from build123d import *

# Parameters (mm, degrees)
EXTRUDE_1_DEPTH        = 52
SKETCH_2_W             = 14.5
SKETCH_2_H             = 8
CUT_EXTRUDE_1_DEPTH    = 4
PATTERN_LINEAR_1_COUNT = 5
PATTERN_LINEAR_1_PITCH = 10
CUT_EXTRUDE_2_DEPTH    = 6.5
PATTERN_LINEAR_2_COUNT = 5
PATTERN_LINEAR_2_PITCH = 10
SKETCH_5_W             = 3
SKETCH_5_H             = 2
SKETCH_5_W_2           = 2
SKETCH_5_H_2           = 1
CUT_EXTRUDE_3_DEPTH    = 3
PATTERN_LINEAR_3_COUNT = 6
PATTERN_LINEAR_3_PITCH = 10
EXTRUDE_2_DEPTH        = 3.5
SKETCH_8_W             = 2
SKETCH_8_H             = 0.5
CUT_EXTRUDE_4_DEPTH    = 5


with BuildPart() as part:
    # 草图1 → 凸台-拉伸1 (new body)
    with BuildSketch(Plane(origin=(0, 0, 0), x_dir=(1, 0, 0), z_dir=(0, 1, 0))):
        Polygon((0, 19), (-2.5, 19), (0, 0), (17.5, 0), (17.5, 3), (3, 3), (3, 19), align=None)
    extrude(amount=EXTRUDE_1_DEPTH)

    # 草图2 → 切除-拉伸1 (cut, through all)
    with BuildSketch(Plane(origin=(0, 0, -3), x_dir=(-1, 0, 0), z_dir=(0, 0, -1))):
        with Locations((-10.25, 46)):
            Rectangle(SKETCH_2_W, SKETCH_2_H)
    cut_extrude_1 = extrude(amount=-CUT_EXTRUDE_1_DEPTH, mode=Mode.SUBTRACT)

    # 阵列(线性)1: 切除-拉伸1 ×5
    with Locations(*[(0, -i * PATTERN_LINEAR_1_PITCH, 0) for i in range(1, PATTERN_LINEAR_1_COUNT)]):
        add(cut_extrude_1, mode=Mode.SUBTRACT)

    # 草图4 → 切除-拉伸2 (cut, through all)
    with BuildSketch(Plane(origin=(3, 0, 0), x_dir=(0, 0, -1), z_dir=(1, 0, 0))):
        Polygon((3, 50), (3, 42), (10, 42.21875), (10, 49.78125), align=None)
        Polygon((19, 49.5), (19, 42.5), (12.5, 42.296875), (12.5, 49.703125), align=None)
    cut_extrude_2 = extrude(amount=-CUT_EXTRUDE_2_DEPTH, mode=Mode.SUBTRACT)

    # 阵列(线性)2: 切除-拉伸2 ×5
    with Locations(*[(0, -i * PATTERN_LINEAR_2_PITCH, 0) for i in range(1, PATTERN_LINEAR_2_COUNT)]):
        add(cut_extrude_2, mode=Mode.SUBTRACT)

    # 草图5 → 切除-拉伸3 (cut)
    with BuildSketch(Plane(origin=(17.5, 0, 0), x_dir=(0, 0, -1), z_dir=(1, 0, 0))):
        with Locations((1.5, 51)):
            Rectangle(SKETCH_5_W, SKETCH_5_H)
        with Locations((1.5, 51)):
            Rectangle(SKETCH_5_W_2, SKETCH_5_H_2, mode=Mode.SUBTRACT)
    cut_extrude_3 = extrude(amount=-CUT_EXTRUDE_3_DEPTH, mode=Mode.SUBTRACT)

    # 阵列(线性)3: 切除-拉伸3 ×6
    with Locations(*[(0, -i * PATTERN_LINEAR_3_PITCH, 0) for i in range(1, PATTERN_LINEAR_3_COUNT)]):
        add(cut_extrude_3, mode=Mode.SUBTRACT)

    # 草图6 → 凸台-拉伸2 (add)
    with BuildSketch(Plane(origin=(3, 0, 0), x_dir=(0, 0, -1), z_dir=(1, 0, 0))):
        Polygon((8.5, 0), (8.5, 0.5), (12.5, 0.5), (12.5, 0), (12.5, -0.5), (8.5, -0.5), align=None)
    extrude_2 = extrude(amount=EXTRUDE_2_DEPTH)

    # 草图8 → 切除-拉伸4 (cut)
    with BuildSketch(Plane.XY.offset(-8.5)):
        with Locations((4, -0.25)):
            Rectangle(SKETCH_8_W, SKETCH_8_H)
        Polygon((6.5, -0.5), (5.1, -0.5), (6.5, 0.2), align=None)
    cut_extrude_4 = extrude(amount=-CUT_EXTRUDE_4_DEPTH, mode=Mode.SUBTRACT)

    # 镜向1: 凸台-拉伸2, 切除-拉伸4 across plane
    add(extrude_2.mirror(Plane.ZX.offset(26)))
    add(cut_extrude_4.mirror(Plane.ZX.offset(26)), mode=Mode.SUBTRACT)


solid = part.part
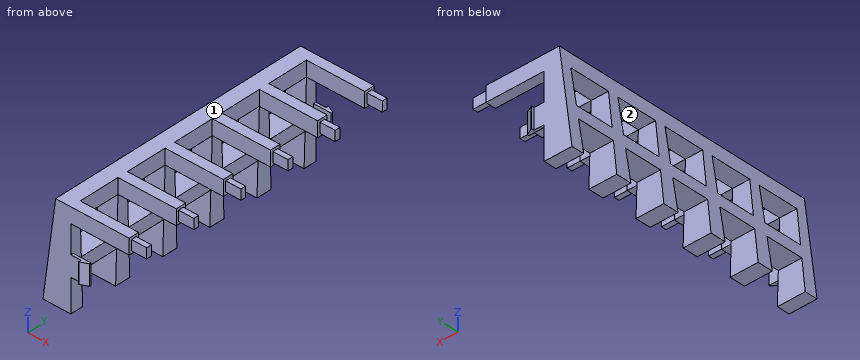
The listing builds one solid part. Answer for the finished solid, in the listing's coordinates (mm). Face numbers are marked on the shaded views. Coordinates: 2 decimals unless noted, no trailing zeros. Order: outer loops, then holes, each group sorted by start corner. A loop starts at its lowest first (then second) coordinate and runs counter-clockwise, first axis right, second up. Notation, with made-up numbers: (-20.5, 81.25) -> (-11.5, 81.25) arc R16 ccw to (-11.5, 89.25) -> close; hole circle Ø6 at (-15, 15). An arc over 180 degrees is marked (long way). Answer in a Markdown table with one row per item. Add a question column.
Item 1: Find section C-C (z = -13.25). Write down the section's boundary in (x, y).
Item 2: Find the intervals of material crossed by L1, parallel to Y at x = 12.75, z = -1.75; L2, parallel to Y at x = 15.5, z = -1.75; L3, parallel to Z at x = 2.25, y = 13, in increasing order. Write a range as from..to.
Item 3: Find section B-B (y = 16). Write down the section's boundary in (x, z).
Item 4: Find section D-D (x = 11). Write down the section's boundary in (y, z).
Item 5: Find section A-A (x = 4.25). State how many separate pieces and enclosed holes the cut face has, then the cut area to 3 significant figures.
Item 6: Determine the mould class of the marked faces 1 and 2 for opening direction Y: +Y half, -Y half, draft (parallel to the pull), parting line (faces both ways), or undercut.
Item 7: Each of these flat-tipped pins is pushed along its axis until it touches: P1, Ø2.5, axis at x = 9.5, z = -1, coming from the -Y side; P2, Ø2, axis at x = 16, z = -1.5, coming from the +Y side; P3, Ø1.6, axis at x = 16, z = -1, coming from the -Y side; P4, Ø2, axis at x = 1.5, y = 25.5, coming from the +Z side. Where does it stop, or does it pass through?
Result set:
| question | item | result |
|---|---|---|
| 1 | outline | (-1.74, 0) -> (3, 0) -> (3, 2.32) -> (-1.74, 2.32) -> close; (-1.74, 9.68) -> (3, 9.68) -> (3, 12.32) -> (-1.74, 12.32) -> close; (-1.74, 19.68) -> (3, 19.68) -> (3, 22.32) -> (-1.74, 22.32) -> close; (-1.74, 29.68) -> (3, 29.68) -> (3, 32.32) -> (-1.74, 32.32) -> close; (-1.74, 39.68) -> (3, 39.68) -> (3, 42.32) -> (-1.74, 42.32) -> close; (-1.74, 49.68) -> (3, 49.68) -> (3, 52) -> (-1.74, 52) -> close |
| 2 | L1 | y = 0..2, 10..12, 20..22, 30..32, 40..42, 50..52 |
| 2 | L2 | y = 0.5..1.5, 10.5..11.5, 20.5..21.5, 30.5..31.5, 40.5..41.5, 50.5..51.5 |
| 2 | L3 | z = -12.5..-10, -3..0 |
| 3 | outline | (-1.64, -12.5) -> (3, -12.5) -> (3, -10) -> (-1.32, -10) -> close; (-0.39, -3) -> (3, -3) -> (3, 0) -> (0, 0) -> close |
| 4 | outline | (0, -3) -> (2, -3) -> (2, 0) -> (0, 0) -> close; (10, -3) -> (12, -3) -> (12, 0) -> (10, 0) -> close; (20, -3) -> (22, -3) -> (22, 0) -> (20, 0) -> close; (30, -3) -> (32, -3) -> (32, 0) -> (30, 0) -> close; (40, -3) -> (42, -3) -> (42, 0) -> (40, 0) -> close; (50, -3) -> (52, -3) -> (52, 0) -> (50, 0) -> close |
| 5 | separate pieces | 8 |
| 5 | enclosed holes | 0 |
| 5 | area | 40.0 mm² |
| 6 | face 1 | draft |
| 6 | face 2 | undercut |
| 7 | P1 | stops at y = 0 |
| 7 | P2 | stops at y = 51.5 |
| 7 | P3 | stops at y = 0.5 |
| 7 | P4 | stops at z = 0 |
